The listing builds one solid part. Answer for the finished solid, in the listing's coordinates (mm). Round coordinates to 2 decimals unless told otherwise and drop trailing zeros. Write each loop counter-clockwise with the first axis right and the second up, starting at its lowest first coordinate (ties: lowest second). Pieces come first, ordered by that corner, then holes.
(1) Each of these flat-tipped pins is pushed along its axis until it touches: pin 1 Ø3.5 at (x, z) = (24, 1.5) entering from -Y; pin 2 Ø1.3 at (x, z) = (-1, 2) entering from -Y; pin 3 Ø0.6 at (x, z) = (2.5, -0.5) entering from +Y. Where does it stop, or does it pass through?
(2) A cutting plane is placed at A-A, the plane x = 0. Give the vertices of the cut face in (y, z), and give its area (3 significant figures).
(3) Find the intervals of material crossed by probe 1 along X at (y, z) = (-39.1, 1.5); probe 2 along Y at (x, z) = (3.5, 4); probe 3 along Y at (x, z) = (-23, 0.75), in increasing order.
(4) A cutting plane is placed at B-B, the plane z = 1.5. Give the vertices of the cut face in (x, y), and give its area (3 significant figures).
(5) A cutting plane is placed at D-D, the plane y = -17.5. Give the vertices of the cut face in (x, z), and give its area (3 significant figures).
(6) A cutting plane is placed at C-C, the plane x = 9. Give the vertices of the cut face in (y, z).
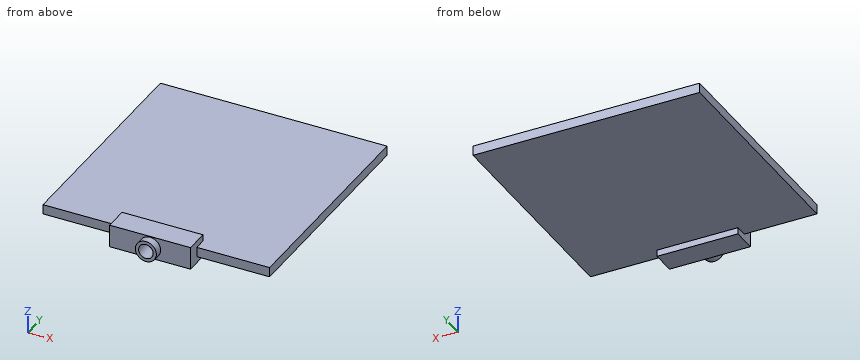
from build123d import *

# Parameters (mm, degrees)
SKETCH1_W                = 70
SKETCH1_H                = 70
BOSS_EXTRUDE1_DEPTH      = 3
BOSS_EXTRUDE2_DEPTH      = 2
BOSS_EXTRUDE2_DEPTH_BACK = 5
SKETCH2_W                = 25
SKETCH2_H                = 7.41284488
SKETCH3_R                = 2.25
CUT_EXTRUDE1_DEPTH       = 2.5
BOSS_EXTRUDE3_START      = 2.5
SKETCH4_R                = 3.25
SKETCH4_R_2              = 2.25
BOSS_EXTRUDE3_DEPTH      = 2.5


with BuildPart() as part:
    # Sketch1 → Boss-Extrude1 (new body)
    with BuildSketch(Plane.XY):
        Rectangle(SKETCH1_W, SKETCH1_H)
    extrude(amount=BOSS_EXTRUDE1_DEPTH)

    # Sketch2 → Boss-Extrude2 (add, two sides: drawn at the far end of the back side and taken through both)
    with BuildSketch(Plane(origin=(0, 0, 0), x_dir=(-1, 0, 0), z_dir=(0, 0, -1)).offset(-BOSS_EXTRUDE2_DEPTH_BACK)):
        with Locations((0, -35)):
            Rectangle(SKETCH2_W, SKETCH2_H)
    extrude(amount=BOSS_EXTRUDE2_DEPTH + BOSS_EXTRUDE2_DEPTH_BACK)

    # Sketch3 → Cut-Extrude1 (cut)
    with BuildSketch(Plane.XZ.offset(38.70642244)):
        with Locations(Location((0, 1.5, 0), (0, 0, 270))):
            Circle(SKETCH3_R)
    extrude(amount=-CUT_EXTRUDE1_DEPTH, mode=Mode.SUBTRACT)

    # Sketch4 → Boss-Extrude3 (add)
    with BuildSketch(Plane.XZ.offset(38.70642244).offset(BOSS_EXTRUDE3_START)):
        with Locations(Location((0, 1.5, 0), (0, 0, 270))):
            Circle(SKETCH4_R)
        with Locations(Location((0, 1.5, 0), (0, 0, 270))):
            Circle(SKETCH4_R_2, mode=Mode.SUBTRACT)
    extrude(amount=-BOSS_EXTRUDE3_DEPTH)


solid = part.part
Solutions:
1. pin 1: stops at y = -35
1. pin 2: stops at y = -36.21
1. pin 3: stops at y = -31.29
2. outline: (-41.21, -1.75) - (-38.71, -1.75) - (-38.71, -2) - (-31.29, -2) - (-31.29, 0) - (35, 0) - (35, 3) - (-31.29, 3) - (-31.29, 5) - (-38.71, 5) - (-38.71, 4.75) - (-41.21, 4.75) - (-41.21, 3.75) - (-36.21, 3.75) - (-36.21, -0.75) - (-41.21, -0.75) - close
2. area: 245 mm2
3. probe 1: x = -3.25 to -2.25, 2.25 to 3.25
3. probe 2: y = -38.71 to -31.29
3. probe 3: y = -35 to 35
4. outline: (-35, -35) - (-12.5, -35) - (-12.5, -38.71) - (-3.25, -38.71) - (-3.25, -41.21) - (-2.25, -41.21) - (-2.25, -36.21) - (2.25, -36.21) - (2.25, -41.21) - (3.25, -41.21) - (3.25, -38.71) - (12.5, -38.71) - (12.5, -35) - (35, -35) - (35, 35) - (-35, 35) - close
4. area: 4,990 mm2
5. outline: (-35, 0) - (35, 0) - (35, 3) - (-35, 3) - close
5. area: 210 mm2
6. outline: (-38.71, -2) - (-31.29, -2) - (-31.29, 0) - (35, 0) - (35, 3) - (-31.29, 3) - (-31.29, 5) - (-38.71, 5) - close
